CAD build for the part. Positions are in the model's coordinates, mm. Coordinates: 2 decimals unless noted, no trailing zeros. Write each loop counter-clockwise with the first axis right and the second up, starting at its lowest first coordinate (ties: lowest second). Pieces come first, ordered by that corner, then holes. Notation, with made-up numbers: M 14,87.5 L 68,87.5 A15 ccw 68,112.5 Z; hole C 1.25,12 d11. An arc over 180 degrees is marked long. Answer as CSV lines item,"result". Start each with the question number.
```python
from build123d import *

# Parameters (mm, degrees)
SKETCH1_R           = 23.6982
SKETCH1_R_2         = 22.225
BOSS_EXTRUDE1_DEPTH = 635
CUT_EXTRUDE2_START  = -28.631769
SKETCH3_W           = 3.175
SKETCH3_H           = 174.625
CUT_EXTRUDE2_DEPTH  = 1.529969
CIRPATTERN4_COUNT   = 3


with BuildPart() as part:
    # Sketch1 → Boss-Extrude1 (new body)
    with BuildSketch(Plane.XY):
        Circle(SKETCH1_R)
        Circle(SKETCH1_R_2, mode=Mode.SUBTRACT)
    extrude(amount=BOSS_EXTRUDE1_DEPTH)

    # Sketch3 → Cut-Extrude2 (cut)
    with BuildSketch(Plane(origin=(0, 50.8, 0), x_dir=(1, 0, 0), z_dir=(0, 1, 0)).offset(CUT_EXTRUDE2_START)):
        with Locations((0, -541.3375)):
            Rectangle(SKETCH3_W, SKETCH3_H)
    cut_extrude2 = extrude(amount=CUT_EXTRUDE2_DEPTH, mode=Mode.SUBTRACT)

    # CirPattern4: Cut-Extrude2 ×3 about axis
    cirpattern4_axis = Axis((0, 0, 0), (0, 0, 1))
    for i in range(1, CIRPATTERN4_COUNT):
        add(cut_extrude2.rotate(cirpattern4_axis, i * 360 / CIRPATTERN4_COUNT), mode=Mode.SUBTRACT)


solid = part.part
```
1) Band-saw the part on C-C, the plane z = 330. List the corners of the cut face in (x, y) (3 decimals), plus the area to 3 significant figures.
2) Two-plate mould, pull along Y, no slides. Class faces 1 (the cylindrical face through (21.199, 6.676, 313.055)), 2 (the cylindrical face through (-5.137, -23.135, 313.055)): pulls with the +Y half, pulls with the -Y half, needs draft (parallel to the pull), parting line crosses it, or undercut.
3) Probe L1, parallel to X at y = 1, z = 377.5; L2, parallel to Y at x = 10.5, z = 381. List the from-to ranges inside material, lowest first. Write a range as [from, to].
4) Band-saw the part on A-A, the plane z = 511. State how many separate pieces and enclosed holes the cut face has, plus the area to 3 significant figures.
5) Band-saw the part on B-B, the plane y = 0. List the corners of the cut face in (x, z) (3 decimals), plus the area to 3 significant figures.
6) Pin check, flat tips, straight feed: P1, Ø3, axis at x = 7, z = 358.5, coming from the -Y side; P2, Ø10, axis at y = 10.5, z = 228.5, coming from the -X side; P3, Ø12, axis at x = 9, z = 114.5, coming from the -Y side. Stop position of each tip, or through.
Result sheet:
1,outline,"C 0,0 d47.396; hole C 0,0 d44.45"
1,area,"213 mm²"
2,face 1,"undercut"
2,face 2,"parting line crosses it"
3,L1,"x = [-23.68, -22.2], [22.2, 23.68]"
3,L2,"y = [-21.25, -19.59], [19.59, 21.25]"
4,separate pieces,"3"
4,enclosed holes,"0"
4,area,"198 mm²"
5,outline,"M -23.698,0 L -22.225,0 L -22.225,635 L -23.698,635 Z; M 22.225,0 L 23.698,0 L 23.698,635 L 22.225,635 Z"
5,area,"1,870 mm²"
6,P1,"stops at y = -23.05"
6,P2,"stops at x = -23.05"
6,P3,"stops at y = -23.51"
